Job drawing, mm, ordinate dimensions from the low corner. One solid piece. A direction names the side the tool comes from. Give positions to 0.01 mm unless a question says otherwise; leave off trailing zeros. Loops run counter-clockwise (first coordinate to the right, second up) from the corner with the lowest first, then second, coordinate; pieces in that order, holes last.
Item 1: Saw through at D-D on z = 256.5. Give the cut face in (x, y).
Item 2: Which spindle directions (+Z, -Z, +X, -X, +Y, -Y) get a long thin tool onto all of the face, cutting with end or side? Do the marked faces 1, 2 and 3. Say none if no direction does.
Item 3: Saw through at C-C on x = 224.5. Give the cut face in (y, z).
Item 4: Drop flat-ended pins along their axis: P1, Ø5, axis at x = 154.5, z = 731.5, coming from the -Y side; P2, Ø1, axis at x = 194.5, y = 212.5, coming from the +Z side; P3, Ø6, axis at x = 295, y = 174, coming from the -Z side; P4, Ø7.5, axis at x = 82.5, z = 933.5, coming from the -Y side. Give the stop position or say it passes through.
Item 5: Mould opens along Z. For the marked faces 4, 5 and 6 say: released by +Z, released by -Z, zero draft, split by the parting line, or undercut.
Item 6: Probe probe 1 along Z at (x, y) = (250, 479.5); probe 2 along Z at (x, y) = (213, 383); probe 3 along X at (y, z) = (230, 1563.5). List the from-to ranges inside material, lowest first.
Item 7: Saw through at A-A on x = 86.5. Give the cut face in (y, z).
Item 8: Saw through at B-B on y = 311. Give the cut face in (x, z).
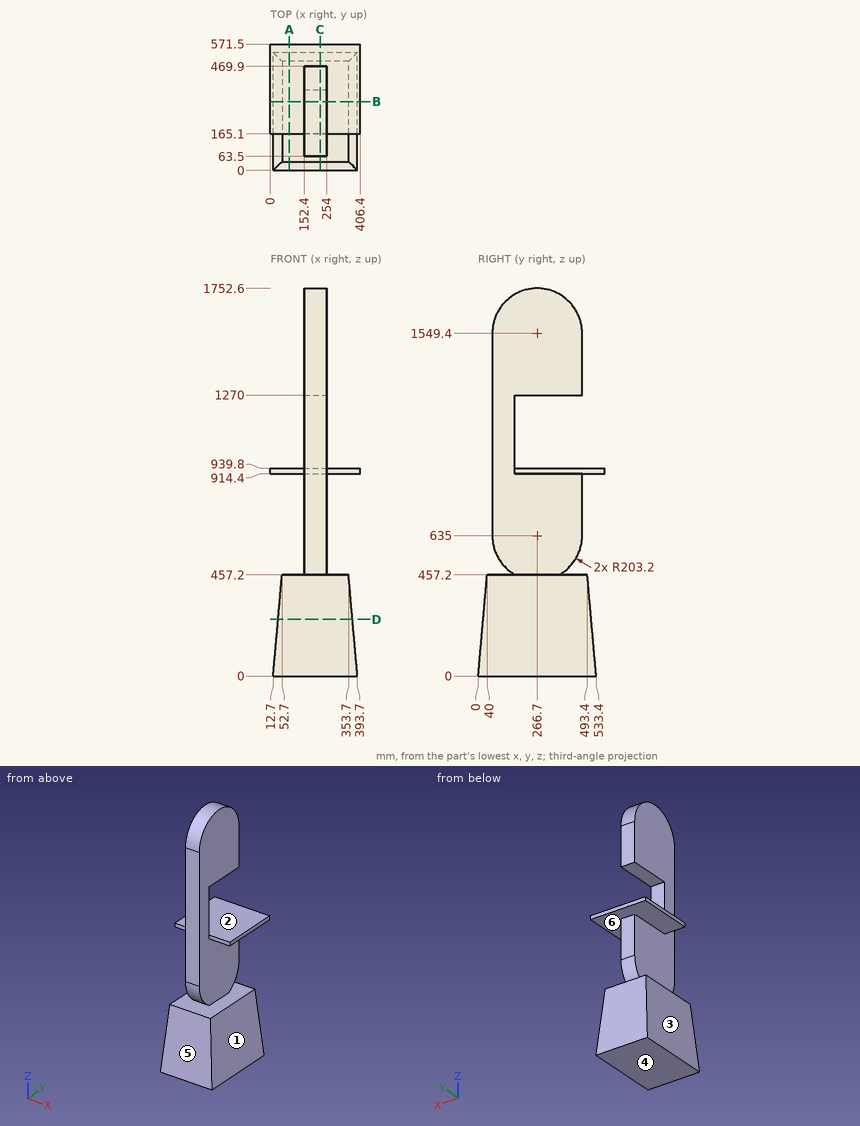
Results below:
1. outline: (35.14, 22.44) - (371.26, 22.44) - (371.26, 510.96) - (35.14, 510.96) - close
2. face 1: +X, +Y, -Y
2. face 2: +X, -X, +Y
2. face 3: -X, +Y, -Y
3. outline: (0, 0) - (533.4, 0) - (493.4, 457.2) - (365.07, 457.2) arc R203.2 ccw to (469.9, 635) - (469.9, 914.4) - (571.5, 914.4) - (571.5, 939.8) - (165.1, 939.8) - (165.1, 1270) - (469.9, 1270) - (469.9, 1549.4) arc R203.2 ccw to (63.5, 1549.4) - (63.5, 635) arc R203.2 ccw to (168.33, 457.2) - (40, 457.2) - close
4. P1: stops at y = 63.5
4. P2: stops at z = 1745.38
4. P3: stops at z = 0
4. P4: stops at y = 165.1
5. face 4: released by -Z
5. face 5: released by +Z
5. face 6: undercut
6. probe 1: z = 0 to 457.2, 914.4 to 939.8
6. probe 2: z = 0 to 457.2, 468.37 to 939.8, 1270 to 1716.03
6. probe 3: x = 152.4 to 254
7. outline: (0, 0) - (533.4, 0) - (493.4, 457.2) - (40, 457.2) - close; (165.1, 914.4) - (571.5, 914.4) - (571.5, 939.8) - (165.1, 939.8) - close
8. outline: (0, 914.4) - (152.4, 914.4) - (152.4, 457.2) - (52.7, 457.2) - (12.7, 0) - (393.7, 0) - (353.7, 457.2) - (254, 457.2) - (254, 914.4) - (406.4, 914.4) - (406.4, 939.8) - (0, 939.8) - close; (152.4, 1270) - (254, 1270) - (254, 1747.71) - (152.4, 1747.71) - close
